Geometry check sheet. Reference: drawing and pictorial views, mm from the part's lowest x, y, z. A direction names the side the tool comes from. Round coordinates to 2 decimals unless told otherwise and drop trailing zeros. Order: outer loops, then holes, each group sorted by start corner. A loop starts at its lowest first (then second) coordinate and runs counter-clockwise, first axis right, second up.
(1) Sectioned sample at B-B, the plane x = 5.5. Enter the section's corners in (y, z), and give its area (3 significant figures).
(2) Sectioned sample at A-A, the plane z = 5.5. Enter the section's corners in (x, y).
(3) Sectioned sample at D-D, the plane y = 3.65. Enter the section's corners in (x, z).
(4) Depth check by flat-ended pin: pin 1 (3 mm diameter, centred on x = 8.5, y = 2, fed in from +Z); pin 2 (2 mm diameter, centred on x = 5, y = 4, fed in from +Z). Enter the tip coordinate at first touch or a pass-through.
(5) Thickness scan on probe 1 along X at (y, z) = (1.8, 9.25); probe 2 along Z at (x, y) = (10.5, 2.5); probe 3 along X at (y, z) = (3.45, 2). Record the ranges inside material, lowest first.
(6) Tool access check on the marked faces 1 and 2. Record the directions out of +Z, -Z, +X, -X, +Y, -Y that give a thin tool (end or side, any length) a straight path to the whole face; none if there is none.
(7) Sectioned sample at C-C, the plane y = 1.8. Enter the section's corners in (x, z), and give its area (3 significant figures).
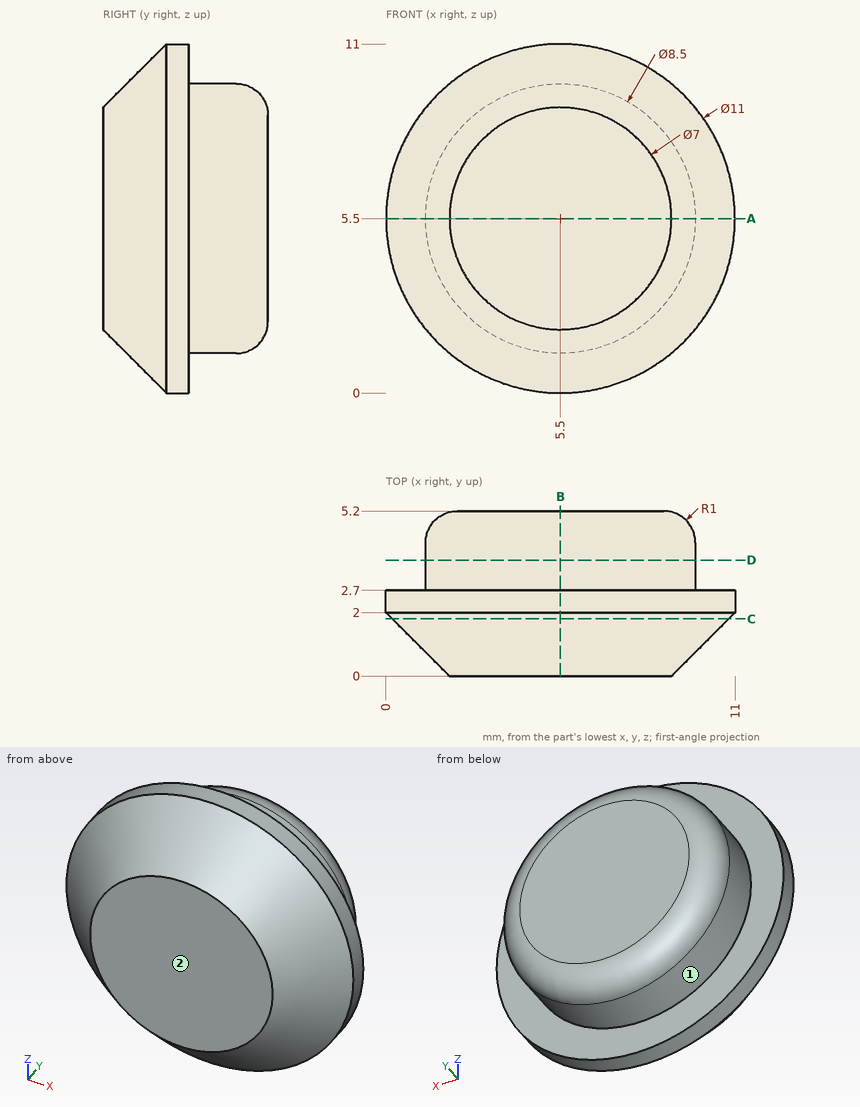
Derived:
1. outline: (0, 2) - (2, 0) - (2.7, 0) - (2.7, 1.25) - (4.2, 1.25) arc R1 ccw to (5.2, 2.25) - (5.2, 8.75) arc R1 ccw to (4.2, 9.75) - (2.7, 9.75) - (2.7, 11) - (2, 11) - (0, 9) - close
1. area: 46.5 mm2
2. outline: (0, 2) - (2, 0) - (9, 0) - (11, 2) - (11, 2.7) - (9.75, 2.7) - (9.75, 4.2) arc R1 ccw to (8.75, 5.2) - (2.25, 5.2) arc R1 ccw to (1.25, 4.2) - (1.25, 2.7) - (0, 2.7) - close
3. outline: circle Ø8.5 at (5.5, 5.5)
4. pin 1: stops at z = 10.79
4. pin 2: stops at z = 9.75
5. probe 1: x = 1.75 to 9.25
5. probe 2: z = 3.21 to 7.79
5. probe 3: x = 3.09 to 7.91
6. face 1: +Y
6. face 2: +Z, -Z, +X, -X, -Y
7. outline: circle Ø10.6 at (5.5, 5.5)
7. area: 88.2 mm2
